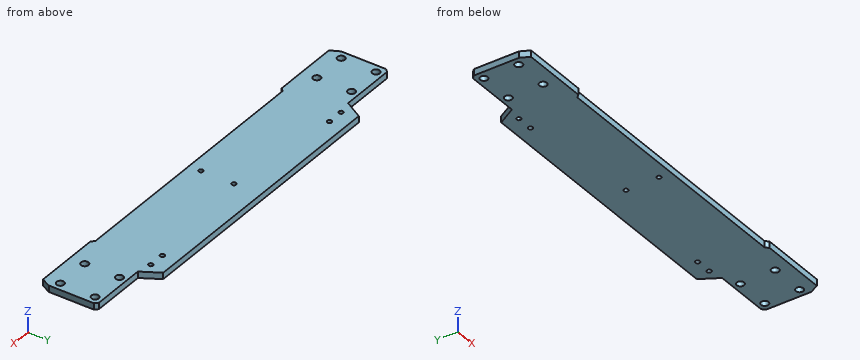
from build123d import *

# Parameters (mm, degrees)
SKETCH1_R           = 2.500025339
SKETCH1_R_2         = 2.500030275
SKETCH1_R_3         = 2.50059385
SKETCH1_R_4         = 2.49996671
SKETCH1_R_5         = 1.500006603
SKETCH1_R_6         = 1.500017827
SKETCH1_R_7         = 1.499993425
SKETCH1_R_8         = 1.500001567
SKETCH1_R_9         = 1.499994017
SKETCH1_R_10        = 2.500046291
SKETCH1_R_11        = 2.500203468
SKETCH1_R_12        = 2.500034464
SKETCH1_R_13        = 2.500151338
BOSS_EXTRUDE1_DEPTH = 4.25


with BuildPart() as part:
    # Sketch1 → Boss-Extrude1 (new body)
    with BuildSketch(Plane.XY):
        Polygon((-89, -1), (89, -1), (91, -3), (136, -3), (139, 3), (139, 33), (137, 35), (100, 35), (93, 47), (-93, 47), (-100, 35), (-137, 35), (-139, 33), (-139, 3), (-136, -3), (-91, -3), align=None)
        with Locations((-133.600349177, 30.099805675)):
            Circle(SKETCH1_R, mode=Mode.SUBTRACT)
        with Locations((-110.397163401, 30.086562155)):
            Circle(SKETCH1_R_2, mode=Mode.SUBTRACT)
        with Locations((-133.597969419, 6.885824912)):
            Circle(SKETCH1_R_3, mode=Mode.SUBTRACT)
        with Locations((-110.4, 6.899985)):
            Circle(SKETCH1_R_4, mode=Mode.SUBTRACT)
        with Locations((-90.5, 37)):
            Circle(SKETCH1_R_5, mode=Mode.SUBTRACT)
        with Locations((-79.435047391, 37.005403238)):
            Circle(SKETCH1_R_6, mode=Mode.SUBTRACT)
        with Locations((1.6217e-05, 29.00002115)):
            Circle(SKETCH1_R_7, mode=Mode.SUBTRACT)
        with Locations((0.007512826, 6.993184051)):
            Circle(SKETCH1_R_8, mode=Mode.SUBTRACT)
        with Locations((79.5, 37)):
            Circle(SKETCH1_R_5, mode=Mode.SUBTRACT)
        with Locations((90.500005983, 37.00001129)):
            Circle(SKETCH1_R_9, mode=Mode.SUBTRACT)
        with Locations((110.399953709, 30.100043687)):
            Circle(SKETCH1_R_10, mode=Mode.SUBTRACT)
        with Locations((133.599796532, 30.099959619)):
            Circle(SKETCH1_R_11, mode=Mode.SUBTRACT)
        with Locations((110.399965537, 6.899913257)):
            Circle(SKETCH1_R_12, mode=Mode.SUBTRACT)
        with Locations((133.599879489, 6.899786711)):
            Circle(SKETCH1_R_13, mode=Mode.SUBTRACT)
    extrude(amount=BOSS_EXTRUDE1_DEPTH)


solid = part.part
Could you check a few things on this model? Use its own coordinates, in mm. Coordinates: 2 decimals unless noted, no trailing zeros. Order: outer loops, then holes, each group sorted by start corner. A loop starts at its lowest first (then second) coordinate and runs counter-clockwise, first axis right, second up.
Q1. Will these pins go through, and if not, where does the flat tip stop? pin 1 (4.5 mm diameter, centred on x = 110.4, y = 30.1, fed in from -Z) (3 decimals); pin 2 (2 mm diameter, centred on x = -110.5, z = 2.5, fed in from +Y); pin 3 (1.5 mm diameter, centred on x = 45, z = 1.5, fed in from -Y).
Q2. Suppose I cut it at A-A on z = 0.75. Give the number of separate pieces and of enclosed holes in the cut face, and give its area (3 significant figures).
Q3. Please list where these lines run through material, in increasing order: L1, parallel to Y at x = -79.5, z = 0.6; L2, parallel to X at y = 36, z = 2.8; L3, parallel to Y at x = 106, z = 0.6.
Q4. Suppose I cut it at B-B on x = -104. Please give me the cut outline in (y, z), and give its area (4 significant figures).
Q5. Suppose I cut it at C-C on x = 59.5. Please give me the cut outline in (y, z).
Answer:
1. pin 1: passes through
1. pin 2: stops at y = 35
1. pin 3: stops at y = -1
2. separate pieces: 1
2. enclosed holes: 14
2. area: 12,300 mm2
3. L1: y = -1 to 35.51, 38.5 to 47
3. L2: x = -99.42 to -91.62, -89.38 to -80.55, -78.32 to 78.38, 80.62 to 89.38, 91.62 to 99.42
3. L3: y = -3 to 35
4. outline: (-3, 0) - (35, 0) - (35, 4.25) - (-3, 4.25) - close
4. area: 161.5 mm2
5. outline: (-1, 0) - (47, 0) - (47, 4.25) - (-1, 4.25) - close
